Design review of the part built by this model. Coordinates are the model's own, in mm. Face numbers are marked on the shaded views. A direction names the side the tool comes from. Give positions to 0.01 mm unless a question says otherwise; leave off trailing zeros. Write each loop counter-clockwise with the first axis right and the second up, starting at its lowest first coordinate (ties: lowest second). Pieces come first, ordered by that corner, then holes. Notation, with made-up numbers: (77, 26) - (136, 26) arc R23 ccw to (136, 46) - close; hole circle Ø11 at (-16.5, 39). An arc over 180 degrees is marked (long way). Write each question's results on one line, items separated by ' | '. Start each with the question number.
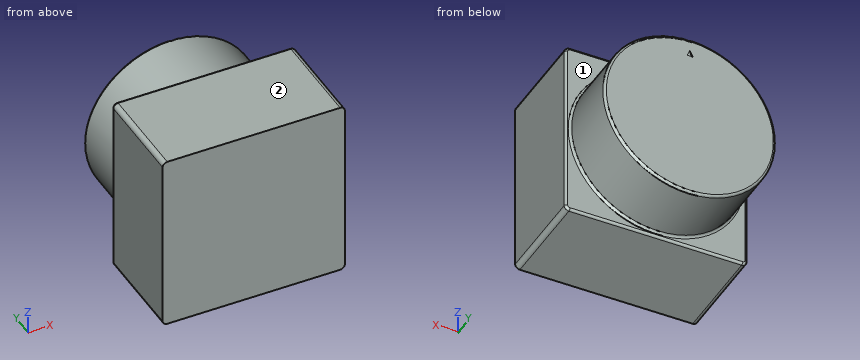
from build123d import *

# Parameters (mm, degrees)
SKETCH_1_W          = 39
SKETCH_1_H          = 39
EXTRUDE_1_DEPTH     = 21
SKETCH_2_R          = 18.38099713
EXTRUDE_2_DEPTH     = 14
FILLET_1_R          = 1
FILLET_2_R          = 0.5
CUT_EXTRUDE_1_DEPTH = 0.1


with BuildPart() as part:
    # 草图1 → 凸台-拉伸1 (new body)
    with BuildSketch(Plane(origin=(0, 0, 0), x_dir=(1, 0, 0), z_dir=(0, 1, 0))):
        Rectangle(SKETCH_1_W, SKETCH_1_H)
    extrude(amount=EXTRUDE_1_DEPTH)

    # 草图2 → 凸台-拉伸2 (add)
    with BuildSketch(Plane(origin=(0, 21, 0), x_dir=(1, 0, 0), z_dir=(0, 1, 0))):
        Circle(SKETCH_2_R)
    extrude(amount=EXTRUDE_2_DEPTH)

    # 圆角1
    fillet_1_edges = [part.edges().sort_by_distance(p)[0] for p in [
        (19.5, 10.5, 19.5),
        (-19.5, 10.5, 19.5),
        (-19.5, 10.5, -19.5),
        (19.5, 10.5, -19.5),
    ]]
    fillet(fillet_1_edges, radius=FILLET_1_R)

    # 圆角2
    fillet_2_edges = [part.edges().sort_by_distance(p)[0] for p in [
        (-18.38099713, 21, 0),
        (-18.38099713, 35, 0),
        (-19.5, 21, 0),
        (0, 21, -19.5),
        (19.5, 21, 0),
        (0, 21, 19.5),
        (19.207106781, 21, -19.207106781),
        (19.207106781, 21, 19.207106781),
        (-19.207106781, 21, 19.207106781),
        (-19.207106781, 21, -19.207106781),
    ]]
    fillet(fillet_2_edges, radius=FILLET_2_R)

    # 草图3 → 切除-拉伸1 (cut)
    with BuildSketch(Plane(origin=(0, 35, 0), x_dir=(1, 0, 0), z_dir=(0, 1, 0))):
        Polygon((0, -15.64459956), (-0.583250004, -14.417555177), (0.583250004, -14.417555177), align=None)
    extrude(amount=-CUT_EXTRUDE_1_DEPTH, mode=Mode.SUBTRACT)


solid = part.part
Q1. Add section B-B on y = 31. State the section outline as (x, z) points.
Q2. For line 1 along Y through (x, z) = (9, 17); line 2 along X through (y, z) = (24.5, 0.5); line 3 along Z through (x, y) = (-15, 27.5), list the stretches that pass through material, from the lowest coordinate up. Write a range as [from, to].
Q3. Add section A-A on z = 0. State the section outline as (x, y) points, plus the area to 3 significant figures.
Q4. Machinability: for the marked faces 1 and 2, which of the approach directions +Z, -Z, +X, -X, +Y, -Y give a long, thin tool a straight path to every point of the face, cutting with its end or side? Answer none if there is none.
Q5. Insertion check: P1, Ø3, axis at y = 23, z = 13.5, coming from the -X side; P2, Ø6, axis at y = 24.5, z = -1.5, coming from the +X side; P3, Ø5, axis at x = 2.5, y = 25.5, coming from the +Z side. Each pin has a flat end and moves straight along its axis. Give the tip position at first contact, or say it passes through.
Result:
1) outline: circle Ø36.76 at (0, 0)
2) line 1: y = [0, 21] | line 2: x = [-18.37, 18.37] | line 3: z = [-10.62, 10.62]
3) outline: (-19.5, 0) - (19.5, 0) - (19.5, 20.5) arc R0.5 ccw to (19, 21) - (18.88, 21) arc R0.5 cw to (18.38, 21.5) - (18.38, 34.5) arc R0.5 ccw to (17.88, 35) - (-17.88, 35) arc R0.5 ccw to (-18.38, 34.5) - (-18.38, 21.5) arc R0.5 cw to (-18.88, 21) - (-19, 21) arc R0.5 ccw to (-19.5, 20.5) - close | area: 1,330 mm²
4) face 1: +Y | face 2: +Z, +X, -X, +Y, -Y
5) P1: stops at x = -13.92 | P2: stops at x = 18.38 | P3: stops at z = 18.38
